Geometry check sheet. Reference: the model listing, model coordinates, mm. Face numbers are marked on the shaded views. A direction names the side the tool comes from. Coordinates: 2 decimals unless noted, no trailing zeros. Answer as a JSON object with one key per item and string values.
from build123d import *

# Parameters (mm, degrees)
F5_R = 20
F4_R = 15


with BuildPart() as f6:
    # F0 (on Top) → F6 section 0
    with BuildSketch(Plane.XY):
        Polygon((60, 0), (30, 51.961524), (-30, 51.961524), (-60, 0), (-30, -51.961524), (30, -51.961524), align=None)
    # F2 (on offset) → F6 section 1
    with BuildSketch(Plane.XY.offset(30)):
        Polygon((40, 0), (20, 34.641016), (-20, 34.641016), (-40, 0), (-20, -34.641016), (20, -34.641016), align=None)
    loft()

    # F5 (on face) → F7 section 0
    with BuildSketch(Plane.XY.offset(30)):
        Circle(F5_R)
    # F4 (on offset) → F7 section 1
    with BuildSketch(Plane.XY.offset(90)):
        Circle(F4_R)
    loft()


solid = f6.part
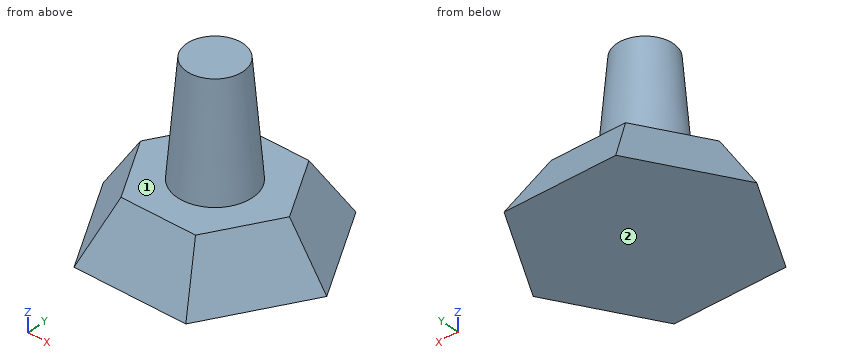
1. Tool access check on the marked faces 1 and 2. Record the directions out of +Z, -Z, +X, -X, +Y, -Y that give a thin tool (end or side, any length) a straight path to the whole face; none if there is none.
Evaluation:
{"face 1": "+Z", "face 2": "-Z, +X, -X, +Y, -Y"}
2. Thickness scan on probe 1 along Z at (x, y) = (-0.5, -23.5); probe 2 along X at (y, z) = (-29.5, 4.5); probe 3 along X at (y, z) = (13, 7). Record the ranges inside material, lowest first. Write a range as from..to.
Evaluation:
{"probe 1": "z = 0..30", "probe 2": "x = -39.97..39.97", "probe 3": "x = -47.83..47.83"}
3. Depth check by flat-ended pin: P1, Ø1, axis at y = -10.5, z = 10.5, coming from the +X side; P2, Ø10, axis at x = 25.5, y = 22.5, coming from the +Z side; P3, Ø12, axis at y = -6, z = 75, coming from the -X side. Enter the tip coordinate at first touch or a pass-through.
Evaluation:
{"P1": "stops at x = 47.38", "P2": "stops at z = 30", "P3": "stops at x = -16.51"}
